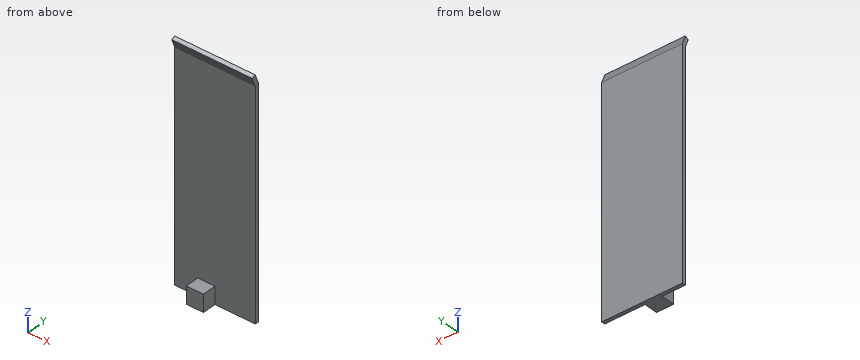
```python
from build123d import *

# Parameters (mm, degrees)
SKETCH1_W                = 6.35
SKETCH1_H                = 6.35
BOSS_EXTRUDE1_DEPTH      = 5.08
BOSS_EXTRUDE2_DEPTH      = 14.850000018
BOSS_EXTRUDE2_DEPTH_BACK = 14.850000018


with BuildPart() as part:
    # Sketch1 → Boss-Extrude1 (new body)
    with BuildSketch(Plane(origin=(0, 0, 0), x_dir=(1, 0, 0), z_dir=(0, 1, 0))):
        Rectangle(SKETCH1_W, SKETCH1_H)
    extrude(amount=BOSS_EXTRUDE1_DEPTH)

    # Sketch2 → Boss-Extrude2 (add, two sides)
    with BuildSketch(Plane(origin=(3.175, 0, 0), x_dir=(0, 0, -1), z_dir=(1, 0, 0))) as boss_extrude2_sk:
        Polygon((3.175, 5.08), (-79.375, 5.08), (-82.741289638, 3.753009016), (-83.26438933, 5.08), (-79.898099692, 6.406990984), (3.175, 6.406990984), align=None)
    extrude(amount=BOSS_EXTRUDE2_DEPTH)
    extrude(boss_extrude2_sk.sketch, amount=-BOSS_EXTRUDE2_DEPTH_BACK)


solid = part.part
```
Verification items for the finished model (mm, model axes). Give positions to 0.01 mm unless a question says otherwise; leave off trailing zeros. Order: outer loops, then holes, each group sorted by start corner. A loop starts at its lowest first (then second) coordinate and runs counter-clockwise, first axis right, second up. Notation, with made-up numbers: (-32, 21) - (18, 21) arc R22 ccw to (18, 50) - close; hole circle Ø7 at (59.5, -2.75). An arc over 180 degrees is marked (long way). Answer as CSV lines item,"result". Start each with the question number.
Item 1: Section check B-B, the plane z = 38.5. Record the boundary of the cut face in (x, y) (3 decimals).
Item 2: Gauge pin test, flat ends, axial feed: pin 1 (1.5 mm diameter, centred on y = 3.5, z = 47, fed in from +X); pin 2 (1 mm diameter, centred on x = -6, z = 63, fed in from -Y); pin 3 (1.5 mm diameter, centred on y = 4, z = 1, fed in from -X) (3 decimals); pin 4 (1.5 mm diameter, centred on y = 3.5, z = -0.5, fed in from +X) (3 decimals). Record the tip position at first contact, or that the pin passes through.
Item 3: Section check D-D, the plane x = 14.75. Record the boundary of the cut face in (y, z) (3 decimals).
Item 4: Section check C-C, the plane y = 1. Record the boundary of the cut face in (x, z) (3 decimals).
Item 5: Material ranges on L1, parallel to Y at x = 4.5, z = 56; L2, parallel to Z at x = 3, y = 3.5 (3 decimals), recorded low to high.
Item 6: Section check A-A, the plane x = 0.5. Record the boundary of the cut face in (y, z) (3 decimals), plus the area to 3 significant figures.
Filled in:
1,outline,"(-11.675, 5.08) - (18.025, 5.08) - (18.025, 6.407) - (-11.675, 6.407) - close"
2,pin 1,"through"
2,pin 2,"y = 5.08"
2,pin 3,"x = -3.175"
2,pin 4,"x = 3.175"
3,outline,"(3.753, 82.741) - (5.08, 79.375) - (5.08, -3.175) - (6.407, -3.175) - (6.407, 79.898) - (5.08, 83.264) - close"
4,outline,"(-3.175, -3.175) - (3.175, -3.175) - (3.175, 3.175) - (-3.175, 3.175) - close"
5,L1,"5.08 to 6.41"
5,L2,"-3.175 to 3.175"
6,outline,"(0, -3.175) - (6.407, -3.175) - (6.407, 79.898) - (5.08, 83.264) - (3.753, 82.741) - (5.08, 79.375) - (5.08, 3.175) - (0, 3.175) - close"
6,area,"147 mm^2"
